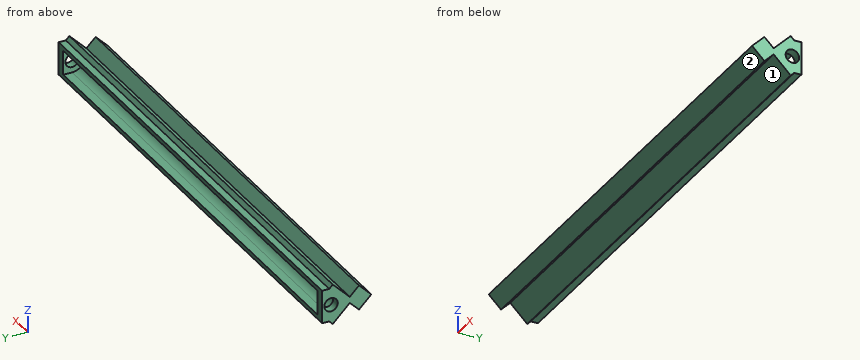
from build123d import *

# Parameters (mm, degrees)
STOCK_PFRD_START               = -138.967906757
STOCK_PFRD_JOINER_BASE_1_DEPTH = 115.804519766
BOSS_EXTRUDE1_DEPTH            = 115.804519766
CUT_EXTRUDE1_START             = -2
SKETCH3_R                      = 1.55
CUT_EXTRUDE1_DEPTH             = 111.804519766
CUT_EXTRUDE2_DEPTH             = 200.295085296
CUT_EXTRUDE2_DEPTH_BACK        = 200.295085296
SKETCH3_2_R                    = 1.55
BOSS_EXTRUDE2_DEPTH            = 2


# Read off the part's stored shape, not the designer's step: Stock-PFRD - Joiner Base-1
with BuildPart() as part:
    # Stock-PFRD - Joiner Base-1 outline → Stock-PFRD - Joiner Base-1 (new body)
    with BuildSketch(Plane.YZ.offset(STOCK_PFRD_START)):
        Polygon((-152.481031246, -3.820121679), (-152.491152925, -3.81), (-152.491152925, 3.81), (-152.481031246, 3.820121679), (-153.274781314, 4.613871747), (-157.18154628, 0.707106781), (-159.302866623, 2.828427125), (-162.131293748, 0), (-159.302866623, -2.828427125), (-157.18154628, -0.707106781), (-153.274781314, -4.613871747), align=None)
    extrude(amount=STOCK_PFRD_JOINER_BASE_1_DEPTH)

    # Sketch2 → Boss-Extrude1 (add)
    with BuildSketch(Plane.ZY.offset(138.967906757)):
        Polygon((3.830243359, -152.491152925), (2.166996747, -150.827906314), (-2.166996747, -150.827906314), (-3.830243359, -152.491152925), (3.81, -152.491152925), align=None)
    extrude(amount=-BOSS_EXTRUDE1_DEPTH)

    # Sketch3 → Cut-Extrude1 (cut)
    with BuildSketch(Plane(origin=(-23.163386991, 0, 0), x_dir=(0, 0, -1), z_dir=(1, 0, 0)).offset(CUT_EXTRUDE1_START)):
        with BuildLine():
            Line((2.8, -150.827906314), (2.8, -152.877906314))
            ThreePointArc((2.8, -152.877906314), (0, -155.677906314), (-2.8, -152.877906314))
            Line((-2.8, -152.877906314), (-2.8, -150.827906314))
            ThreePointArc((-2.8, -150.827906314), (0, -148.027906314), (2.8, -150.827906314))
        make_face()
        with Locations(Location((0, -152.877906314, 0), (0, 0, 90))):
            Circle(SKETCH3_R, mode=Mode.SUBTRACT)
    extrude(amount=-CUT_EXTRUDE1_DEPTH, mode=Mode.SUBTRACT)

    # Sketch3<2> → Cut-Extrude2 (cut, two sides: drawn at the far end of the back side and taken through both)
    with BuildSketch(Plane(origin=(-23.163386991, 0, 0), x_dir=(0, 0, -1), z_dir=(1, 0, 0)).offset(-CUT_EXTRUDE2_DEPTH_BACK)):
        with Locations(Location((0, -152.877906314, 0), (0, 0, 90))):
            Circle(SKETCH3_2_R)
    extrude(amount=CUT_EXTRUDE2_DEPTH + CUT_EXTRUDE2_DEPTH_BACK, mode=Mode.SUBTRACT)

    # Sketch4 → Boss-Extrude2 (add)
    with BuildSketch(Plane(origin=(0, -150.827906314, 0), x_dir=(1, 0, 0), z_dir=(0, 1, 0))):
        Polygon((-138.967906757, 2.166996747), (-136.967906757, 2.166996747), (-136.967906757, 2.8), (-25.163386991, 2.8), (-25.163386991, 2.166996747), (-23.163386991, 2.166996747), (-23.163386991, 3.8), (-138.967906757, 3.8), align=None)
    boss_extrude2 = extrude(amount=-BOSS_EXTRUDE2_DEPTH)

    # Mirror1: Boss-Extrude2 across plane
    add(boss_extrude2.mirror(Plane(origin=(0, 0, 0), x_dir=(1, 0, 0), z_dir=(0, 0, -1))))


solid = part.part
Design review of the part built by this model. Coordinates are the model's own, in mm. Face numbers are marked on the shaded views. Round coordinates to 2 decimals unless told otherwise and drop trailing zeros. Loops run counter-clockwise (first coordinate to the right, second up) from the corner with the lowest first, then second, coordinate; pieces in that order, holes last. Notation, with made-up numbers: M 46.5,68.5 L 91.5,68.5 A32 cw 91.5,103.5 Z; hole C 36.5,39 d6. An arc over 180 degrees is marked long. Answer as a JSON object with one key per item and string values.
Item 1: The part is to be moulded in two halves that separate along Y. For the marked faces 1 and 2, say which applies: pulls with the +Y half, pulls with the -Y half, needs draft (parallel to the pull), parting line crosses it, or undercut.
Answer sheet:
{"face 1": "undercut", "face 2": "pulls with the -Y half"}
Item 2: We need section A-A on x = -119. Give the boundary of the cut face in (y, z), and give its area (3 significant figures).
Answer sheet:
{"outline": "M -162.13,0 L -159.3,-2.83 L -157.18,-0.71 L -153.27,-4.61 L -152.46,-3.8 L -150.83,-3.8 L -150.83,-2.8 L -152.88,-2.8 A2.8 cw -152.88,2.8 L -150.83,2.8 L -150.83,3.8 L -152.46,3.8 L -153.27,4.61 L -157.18,0.71 L -159.3,2.83 Z", "area": "31.8 mm^2"}
Item 3: Wall thickness on L1, parallel to Y at x = -138.05, z = 0; L2, parallel to Z at x = -91.5, y = -151.25; L3, parallel to X at y = -154.5, z = 1: over which ranges is each line inside the solid? List them lowest first. Write a range as from..to.
Answer sheet:
{"L1": "y = -162.13..-154.43, -151.33..-150.83", "L2": "z = -3.8..-2.8, 2.8..3.8", "L3": "x = -138.97..-136.97, -25.16..-23.16"}
Item 4: Clearance check with flat-ended pins moving along their axes: P1, Ø2, axis at x = -75.5, z = -1.5, coming from the -Y side; P2, Ø4, axis at y = -152.88, z = 0, coming from the +X side; P3, Ø1, axis at x = -90, y = -151.5, coming from the -Z side; P4, Ø1.3, axis at x = -58, y = -152, coming from the -Z side. State where each tip first meets the part, or that it passes through.
Answer sheet:
{"P1": "stops at y = -161.63", "P2": "stops at x = -23.16", "P3": "stops at z = -3.8", "P4": "stops at z = -3.99"}
